Read the model definition and answer for the solid it produces. Units are mm, in the model's axes. Coordinates: 2 decimals unless noted, no trailing zeros. Write each loop counter-clockwise with the first axis right and the second up, starting at its lowest first coordinate (ties: lowest second). Pieces come first, ordered by that corner, then holes. Notation, with made-up numbers: (36.5, 72) - (45.5, 72) arc R31 ccw to (45.5, 104) - close; hole circle Ø11 at (38.5, 61). An arc over 180 degrees is marked (long way). Use a Markdown table: item, result.
from build123d import *

# Parameters (mm, degrees)
SKETCH_R          = 32.5
PAD_DEPTH         = 8
SKETCH001_R       = 37.5
PAD001_DEPTH      = 3
SKETCH002_R       = 2.25
POCKET_DEPTH      = 3.001
POCKET_DEPTH_BACK = -8.001


with BuildPart() as part:
    # Sketch → Pad (new body)
    with BuildSketch(Plane.XY):
        Circle(SKETCH_R)
    extrude(amount=PAD_DEPTH)

    # Sketch001 → Pad001 (join)
    with BuildSketch(Plane.XY):
        Circle(SKETCH001_R)
    extrude(amount=-PAD001_DEPTH)

    # Sketch002 → Pocket (cut, two sides)
    with BuildSketch(Plane.XY) as pocket_sk:
        with Locations((-15, 0)):
            Circle(SKETCH002_R)
        with Locations((15, 0)):
            Circle(SKETCH002_R)
    extrude(amount=-POCKET_DEPTH, mode=Mode.SUBTRACT)
    extrude(pocket_sk.sketch, amount=-POCKET_DEPTH_BACK, mode=Mode.SUBTRACT)


solid = part.part
(1) A cutting plane is placed at D-D, the plane z = 2.75. Write down the section's boundary in (x, y), and give its area (3 significant figures).
Report:
| item | result |
|---|---|
| outline | circle Ø65 at (0, 0); hole circle Ø4.5 at (-15, 0); hole circle Ø4.5 at (15, 0) |
| area | 3,290 mm² |
(2) Each of these flat-tipped pins is pushed along its axis until it touches: P1, Ø2, axis at y = -8.5, z = 1.5, coming from the -X side; P2, Ø6, axis at y = 17, z = -0.5, coming from the +X side; P3, Ø1.5, axis at y = 23, z = 6.5, coming from the -X side; P4, Ø3.5, axis at x = -15, y = 0, coming from the +Z side. Where does it stop, or does it pass through?
Report:
| item | result |
|---|---|
| P1 | stops at x = -31.62 |
| P2 | stops at x = 34.79 |
| P3 | stops at x = -23.69 |
| P4 | passes through |
(3) Straight lines are drawn through the part: L1, parallel to Z at x = -28.5, y = -21.5; L2, parallel to Y at x = -15.5, z = 0.5; L3, parallel to Y at x = -15, z = 1.75. For each, find the intervals that lie inside material, in ascending order.
Report:
| item | result |
|---|---|
| L1 | z = -3 to 0 |
| L2 | y = -28.57 to -2.19, 2.19 to 28.57 |
| L3 | y = -28.83 to -2.25, 2.25 to 28.83 |
(4) A cutting plane is placed at B-B, the plane x = 0. Write down the section's boundary in (y, z), and give its area (3 significant figures).
Report:
| item | result |
|---|---|
| outline | (-37.5, -3) - (37.5, -3) - (37.5, 0) - (32.5, 0) - (32.5, 8) - (-32.5, 8) - (-32.5, 0) - (-37.5, 0) - close |
| area | 745 mm² |
(5) The mould has two halves that part along Y. Classify faces 1 (the flat face through (-11, 31, 0)), 2 (the cylindrical face through (17.146, 0.676, 2.577)), 3 (the cylindrical face through (31, 9.76, 3.94)): pulls with the +Y half, pulls with the -Y half, needs draft (parallel to the pull), parting line crosses it, or undercut.
Report:
| item | result |
|---|---|
| face 1 | needs draft |
| face 2 | undercut |
| face 3 | parting line crosses it |
(6) A cutting plane is placed at A-A, the plane y = 0. Write down the section's boundary in (x, z).
Report:
| item | result |
|---|---|
| outline | (-37.5, -3) - (-17.25, -3) - (-17.25, 8) - (-32.5, 8) - (-32.5, 0) - (-37.5, 0) - close; (-12.75, -3) - (12.75, -3) - (12.75, 8) - (-12.75, 8) - close; (17.25, -3) - (37.5, -3) - (37.5, 0) - (32.5, 0) - (32.5, 8) - (17.25, 8) - close |
(7) A cutting plane is placed at C-C, the plane x = 15. Write down the section's boundary in (y, z), and give its area (3 significant figures).
Report:
| item | result |
|---|---|
| outline | (-34.37, -3) - (-2.25, -3) - (-2.25, 8) - (-28.83, 8) - (-28.83, 0) - (-34.37, 0) - close; (2.25, -3) - (34.37, -3) - (34.37, 0) - (28.83, 0) - (28.83, 8) - (2.25, 8) - close |
| area | 618 mm² |
